Study the drawing (mm; zero at the part's minimum x, y, z) and answer. A direction names the side the tool comes from. Give positions to 0.01 mm unless a question says otherwise; leave off trailing zeros. Order: outer loops, then holes, each group sorted by start corner. A loop starts at its lowest first (then second) coordinate and runs counter-clockwise, first axis right, second up. Notation, with made-up numbers: (-10, -26.5) - (40, -26.5) arc R13 cw to (40, -14.5) - close; hole circle Ø7 at (34.5, -13.75). An arc over 180 degrees is marked (long way). Write each question's results on one line, items separated by ' | '. Start each with the question number.
1. Section A-A (x = 27.5) is taken. Give the vertices of the cut face in (y, z) (1 decimal).
2. Which of the six approach directions +Z, -Z, +X, -X, +Y, -Y give full straight-line access (tool end or side, diameter ignored) to the marked faces 5, 6, 7 and 8?
3. Determine the mould class of the marked faces 1, 2, 3 and 4 for opening direction Z: released by +Z, released by -Z, zero draft, split by the parting line, or undercut.
4. Flat-ended cylindrical pins translate along their axes: pin 1 (2 mm diameter, centred on x = 19.5, z = 67.5, fed in from -Y) (3 decimals); pin 2 (2 mm diameter, centred on y = 2, z = 55, fed in from +X); pin 3 (5 mm diameter, centred on x = 58, z = 84, fed in from +Y) (3 decimals). Find the tip coordinate at first contact, or state that the pin passes through.
5. Section C-C (z = 61) is taken. Give the vertices of the cut face in (x, y) (1 decimal).
6. Section B-B (y = 18.5) is taken. Give the vertices of the cut face in (x, z) (1 decimal), and give its area (3 significant figures).
7. Find the intervals of material crossed by L1, parallel to X at y = 72, z = 71; L2, parallel to Y at x = 73.5, z = 45; L3, parallel to Z at x = 36, y = 64.5, in increasing order.
8. Section D-D (z = 14) is taken. Give the vertices of the cut face in (x, y) (1 decimal).
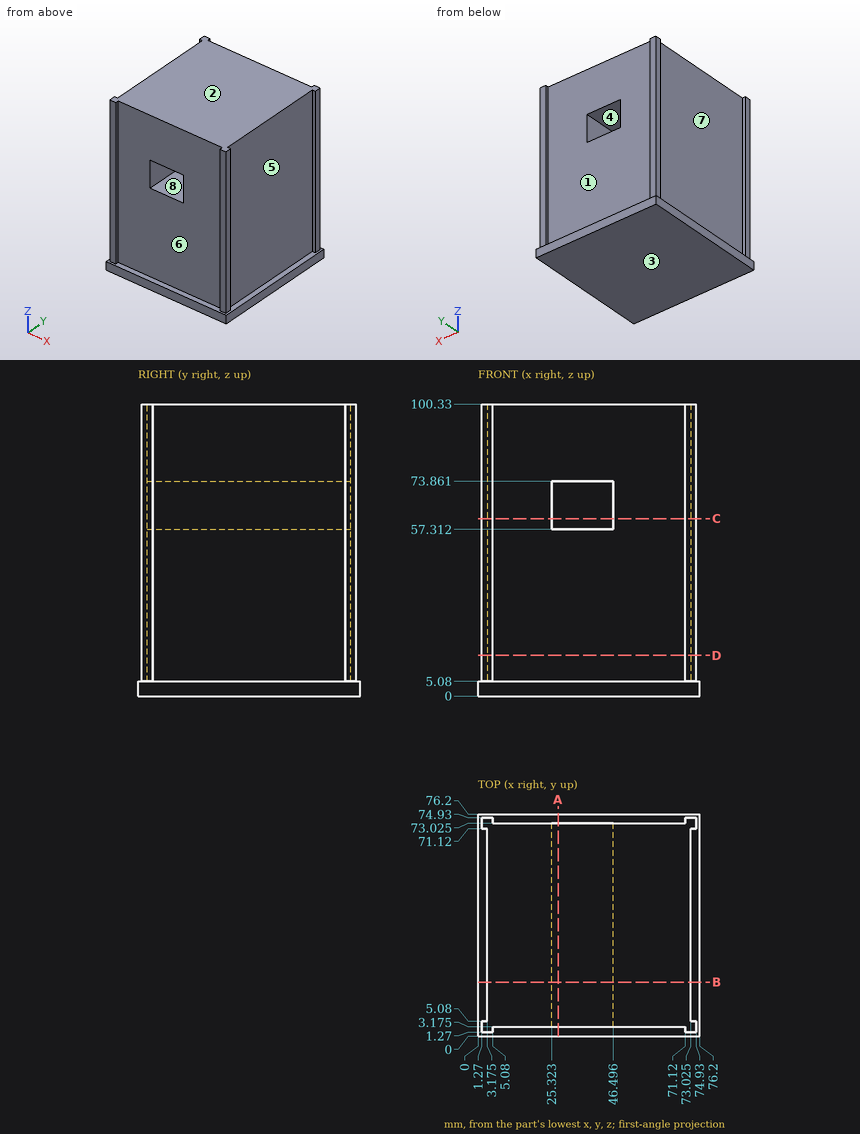
Reported:
1) outline: (0, 0) - (76.2, 0) - (76.2, 5.1) - (73, 5.1) - (73, 57.3) - (3.2, 57.3) - (3.2, 5.1) - (0, 5.1) - close; (3.2, 73.9) - (73, 73.9) - (73, 100.3) - (3.2, 100.3) - close
2) face 5: +Z, +X | face 6: +Z, -Y | face 7: +Z, -X | face 8: +Y, -Y
3) face 1: zero draft | face 2: released by +Z | face 3: released by -Z | face 4: undercut
4) pin 1: y = 3.175 | pin 2: x = 74.93 | pin 3: y = 73.025
5) outline: (1.3, 1.3) - (5.1, 1.3) - (5.1, 3.2) - (25.3, 3.2) - (25.3, 73) - (5.1, 73) - (5.1, 74.9) - (1.3, 74.9) - (1.3, 71.1) - (3.2, 71.1) - (3.2, 5.1) - (1.3, 5.1) - close; (46.5, 3.2) - (71.1, 3.2) - (71.1, 1.3) - (74.9, 1.3) - (74.9, 5.1) - (73, 5.1) - (73, 71.1) - (74.9, 71.1) - (74.9, 74.9) - (71.1, 74.9) - (71.1, 73) - (46.5, 73) - close
6) outline: (0, 0) - (76.2, 0) - (76.2, 5.1) - (73, 5.1) - (73, 100.3) - (3.2, 100.3) - (3.2, 5.1) - (0, 5.1) - close; hole (25.3, 57.3) - (46.5, 57.3) - (46.5, 73.9) - (25.3, 73.9) - close | area: 6,690 mm²
7) L1: 1.27 to 25.32, 46.5 to 74.93 | L2: 1.27 to 5.08, 71.12 to 74.93 | L3: 0 to 57.31, 73.86 to 100.33
8) outline: (1.3, 1.3) - (5.1, 1.3) - (5.1, 3.2) - (71.1, 3.2) - (71.1, 1.3) - (74.9, 1.3) - (74.9, 5.1) - (73, 5.1) - (73, 71.1) - (74.9, 71.1) - (74.9, 74.9) - (71.1, 74.9) - (71.1, 73) - (5.1, 73) - (5.1, 74.9) - (1.3, 74.9) - (1.3, 71.1) - (3.2, 71.1) - (3.2, 5.1) - (1.3, 5.1) - close
